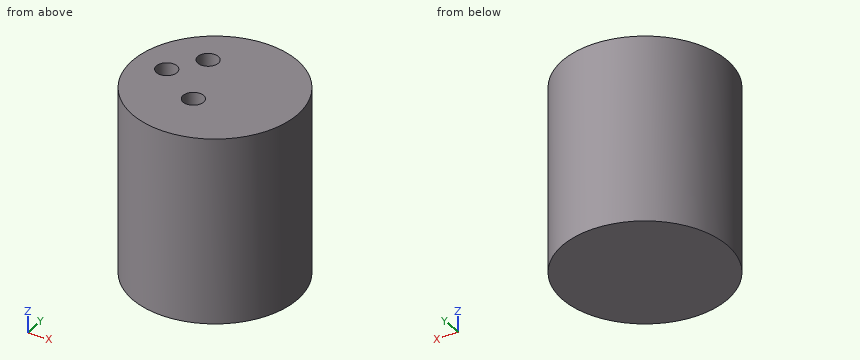
```python
from build123d import *

# Parameters (mm, degrees)
F0_R     = 25.4
F2_DEPTH = 57.15
F4_D     = 6.35
F4_DEPTH = 12.7
F4_TIP   = 1.9077324654


with BuildPart() as f2:
    # F0 (on Top) → F2 (new body, through all)
    with BuildSketch(Plane.XY):
        Circle(F0_R)
    extrude(amount=F2_DEPTH)

    # F4
    with Locations(Plane.XY.offset(57.15)):
        with Locations((-8.8469870389, 10.5592897162), (-15.5139854178, 0.8681075997), (-1.8198583275, -7.7013894916)):
            Hole(F4_D / 2, depth=F4_DEPTH)
            with Locations((0, 0, -(F4_DEPTH + F4_TIP / 2))):  # 118° drill point
                Cone(0, F4_D / 2, F4_TIP, mode=Mode.SUBTRACT)


solid = f2.part
```
Here's how the part is built. I have some questions about the finished solid (model axes, mm). Give positions to 0.01 mm unless a question says otherwise; leave off trailing zeros. Write each loop counter-clockwise with the first axis right and the second up, starting at its lowest first coordinate (ties: lowest second). Pieces come first, ordered by that corner, then holes.
(1) Imagine slicing it at A-A, the plane z = 25. Write out the boundary of the cut face in (x, y), and give its area (3 significant figures).
Output values:
outline: circle Ø50.8 at (0, 0)
area: 2,030 mm2
(2) Imagine slicing it at B-B, the plane x = 18. Write out the boundary of the cut face in (y, z).
Output values:
outline: (-17.92, 0) - (17.92, 0) - (17.92, 57.15) - (-17.92, 57.15) - close
(3) If I drill on L1, parallel to X at y = -0.5, z = 47.5; L2, parallel to X at y = 22, z = 15; L3, parallel to Y at x = 20, z = 8, over which ranges is the centre line in solid material (lowest first)?
Output values:
L1: x = -25.4 to -18.38, -12.65 to 25.4
L2: x = -12.69 to 12.69
L3: y = -15.66 to 15.66
(4) Will these pins go through, and if not, where does the flat tip stop? pin 1 (1 mm diameter, centred on x = 12.5, z = 8, fed in from +Y); pin 2 (8 mm diameter, centred on x = 16.5, y = -4.5, fed in from -Z); pin 3 (8 mm diameter, centred on y = -4.5, z = 6, fed in from -X); pin 4 (2 mm diameter, centred on y = -18.5, z = 24.5, fed in from +X).
Output values:
pin 1: stops at y = 22.39
pin 2: stops at z = 0
pin 3: stops at x = -25.4
pin 4: stops at x = 18.41
